The listing builds one solid part. Answer for the finished solid, in the listing's coordinates (mm). A direction names the side the tool comes from. Coordinates: 2 decimals unless noted, no trailing zeros. Write each loop counter-clockwise with the first axis right and the second up, starting at its lowest first coordinate (ties: lowest second). Pieces come first, ordered by that corner, then holes. Notation, with made-up numbers: M 42,33.5 L 87,33.5 A34 ccw 87,70.5 Z; hole C 75,73.5 d3. An arc over 180 degrees is marked long. Answer as a JSON object with one key per item and string values. Group by question number.
from build123d import *

# Parameters (mm, degrees)
BOSS_EXTRUDE1_DEPTH = 6.35
SKETCH2_R           = 3.175
BOSS_EXTRUDE2_DEPTH = 20.32
SKETCH3_R           = 5.08
BOSS_EXTRUDE3_DEPTH = 2.54


with BuildPart() as part:
    # Sketch1 → Boss-Extrude1 (new body)
    with BuildSketch(Plane.XY):
        with BuildLine():
            Line((0, 5.715), (25.4, 5.715))
            ThreePointArc((25.4, 5.715), (31.115, 0), (25.4, -5.715))
            Line((25.4, -5.715), (0, -5.715))
            ThreePointArc((0, -5.715), (-5.715, 0), (0, 5.715))
        make_face()
    extrude(amount=BOSS_EXTRUDE1_DEPTH)

    # Sketch2 → Boss-Extrude2 (add)
    with BuildSketch(Plane.XY.offset(6.35)):
        with Locations(Location((0, 0, 0), (0, 0, 180))):
            Circle(SKETCH2_R)
    extrude(amount=BOSS_EXTRUDE2_DEPTH)

    # Sketch3 → Boss-Extrude3 (add)
    with BuildSketch(Plane.XY.offset(26.67)):
        Circle(SKETCH3_R)
    extrude(amount=-BOSS_EXTRUDE3_DEPTH)


solid = part.part
Item 1: A tool of negligible diameter and unlimited length cuts with its end or side. For faces 1 (the face through (-0.661, 5.037, 25.418)), 2 (the face through (3.3, -1.1, 24.13)), 3 (the face through (0, 0, 26.67)), from which of +Z, -Z, +X, -X, +Y, -Y can it reach the whole face along a straight path? Write none if from no direction.
Item 2: A cutting plane is placed at D-D, the plane y = -4. Write down the section's boundary in (x, z), and give its area (3 significant figures).
Item 3: A cutting plane is placed at B-B, the plane x = 2.5. Write down the section's boundary in (y, z) (3 decimals), and give its area (3 significant figures).
Item 4: A cutting plane is placed at A-A, the plane y = 0. Write down the section's boundary in (x, z) (3 decimals), and give its area (3 significant figures).
Item 5: Flat-ended cylindrical pins translate along their axes: pin 1 Ø5.5 at (x, y) = (8, -2.5) entering from +Z; pin 2 Ø1 at (y, z) = (3.5, 3) entering from -X; pin 3 Ø4 at (y, z) = (-2.5, 10) entering from -X. Find the tip coordinate at first contact, or state that the pin passes through.
Item 6: A cutting plane is placed at C-C, the plane z = 3.5. Write down the section's boundary in (x, y) (3 decimals), and give its area (3 significant figures).
Item 7: Consider L1, parallel to Z at x = -1, y = -3.5; L2, parallel to Z at x = 28.5, y = -2.75; L3, parallel to X at y = 2.5, z = 5. Determine where each line is inside the solid, lowest interval first. Write a range as from..to.
Answer:
{
 "1": {"face 1": "+Z", "face 2": "none", "face 3": "+Z, +X, -X, +Y, -Y"},
 "2": {"outline": "M -4.08,0 L 29.48,0 L 29.48,6.35 L -4.08,6.35 Z; M -3.13,24.13 L 3.13,24.13 L 3.13,26.67 L -3.13,26.67 Z", "area": "229 mm2"},
 "3": {"outline": "M -5.715,0 L 5.715,0 L 5.715,6.35 L 1.957,6.35 L 1.957,24.13 L 4.422,24.13 L 4.422,26.67 L -4.422,26.67 L -4.422,24.13 L -1.957,24.13 L -1.957,6.35 L -5.715,6.35 Z", "area": "165 mm2"},
 "4": {"outline": "M -5.715,0 L 31.115,0 L 31.115,6.35 L 3.175,6.35 L 3.175,24.13 L 5.08,24.13 L 5.08,26.67 L -5.08,26.67 L -5.08,24.13 L -3.175,24.13 L -3.175,6.35 L -5.715,6.35 Z", "area": "373 mm2"},
 "5": {"pin 1": "z = 6.35", "pin 2": "x = -4.86", "pin 3": "x = -3.14"},
 "6": {"outline": "M 0,-5.715 L 25.4,-5.715 A5.715 ccw 25.4,5.715 L 0,5.715 A5.715 ccw Z", "area": "393 mm2"},
 "7": {"L1": "0..6.35, 24.13..26.67", "L2": "0..6.35", "L3": "-5.14..30.54"}
}
